Solid Edge part; units mm, degrees
sketch "Sketch1" plane through (0, 0, 0) normal (0, 0, 1) x (1, 0, 0)
  line L0 (2.0207, -3.5) -> (4.0415, 0)
  line L1 (4.0415, 0) -> (2.0207, 3.5)
  line L2 (2.0207, 3.5) -> (-2.0207, 3.5)
  line L3 (-2.0207, 3.5) -> (-4.0415, 0)
  line L4 (-4.0415, 0) -> (-2.0207, -3.5)
  line L5 (-2.0207, -3.5) -> (2.0207, -3.5)
extrude "Protrusion1" add sketch "Sketch1" against normal blind 2.5
sketch "Sketch2" plane through (0, 0, 0) normal (0, -1, 0) x (1, 0, 0)
  line L0 (3.5, 0) -> (4.0415, -0.3125)
  line L1 (4.0415, -0.3125) -> (4.0415, 0)
  line L2 (4.0415, 0) -> (3.5, 0)
revolve "RevolvedCutout1" cut sketch "Sketch2" angle 360 about axis through (0, 0, 0.6231) along (0, 0, -1)
sketch "Sketch3" plane through (0, 0, -2.5) normal (0, 0, -1) x (0.5, 0.866, 0)
  circle A0 centre (0, 0) radius 5
extrude "ExtrudedProtrusion_2" add sketch "Sketch3" along normal blind 0.5
sketch "Sketch4" plane through (0, 0, 0) normal (0, 0, 1) x (1, 0, 0)
  circle A0 centre (0, 0) radius 3.5
extrude "ExtrudedProtrusion_3" add sketch "Sketch4" against normal blind 10
For this review, take the finished solid that the model builds, in its own axes (mm). A direction names the side the tool comes from. Coordinates: 2 decimals unless noted, no trailing zeros. Write each loop counter-clockwise with the first axis right and the second up, starting at its lowest first coordinate (ties: lowest second). Pieces come first, ordered by that corner, then holes. Notation, with made-up numbers: (-32, 66.5) - (12, 66.5) arc R11 cw to (12, 71.5) - close; hole circle Ø7 at (70, 72). An arc over 180 degrees is marked (long way). Put each result on its own line as item: value.
1. Add section B-B, the plane z = -9. Give the boundary of the cut face in (x, y).
Values found:
outline: circle Ø7 at (0, 0)
2. Machinability: for faces 1 (the flat face through (-3, 1.8, -1.2)), 2 (the flat face through (-2.2, -3.3, -3)), 3 (the flat face through (0, -3.5, -1)), which of the approach directions +Z, -Z, +X, -X, +Y, -Y give a long, thin tool a straight path to every point of the face, cutting with its end or side? Answer none if there is none.
Values found:
face 1: +Z, -X, +Y
face 2: -Z
face 3: +Z, +X, -X, -Y
3. For pin 1 (3 mm diameter, centred on x = 1, y = 0.5, fed in from +Z); pin 2 (2 mm diameter, centred on x = -0.5, z = -1, fed in from -Y); pin 3 (6 mm diameter, centred on y = -0.5, z = -7, fed in from -X); pin 4 (6 mm diameter, centred on y = 1.5, z = -8, fed in from +X), all flat-tipped, find the tip position at first contact; note any pin that passes through.
Values found:
pin 1: z = 0
pin 2: y = -3.5
pin 3: x = -3.5
pin 4: x = 3.5
4. Wall thickness on probe 1 along Z at (x, y) = (-4.5, -0.25); probe 2 along X at (y, z) = (-0.5, -6.75); probe 3 along Y at (x, z) = (-2, -4.25): over which ranges is each line inside the solid? List them lowest first.
Values found:
probe 1: -3 to -2.5
probe 2: -3.46 to 3.46
probe 3: -2.87 to 2.87
5. Add section A-A, the plane z = -2.25. Give the boundary of the cut face in (x, y).
Values found:
outline: (-4.04, 0) - (-2.02, -3.5) - (2.02, -3.5) - (4.04, 0) - (2.02, 3.5) - (-2.02, 3.5) - close
